```python
from build123d import *

# Parameters (mm, degrees)
BOSS_EXTRUDE1_DEPTH = 42
BOSS_EXTRUDE2_DEPTH = 1
BOSS_EXTRUDE3_DEPTH = 13


with BuildPart() as part:
    # Sketch1 → Boss-Extrude1 (new body)
    with BuildSketch(Plane(origin=(0, 0, 0), x_dir=(0, 0, -1), z_dir=(1, 0, 0))):
        Polygon((0, 4.2), (0, 0), (10.9, 0), (10.9, 0.81375), (1, 0.81375), (1, 1.91375), (0.9, 1.91375), (0.9, 3.2), (1, 3.2), (1, 4.2), align=None)
        Polygon((10.9, 0.81375), (10.9, 0), (21.8, 0), (21.8, 4.2), (20.8, 4.2), (20.8, 3.2), (20.9, 3.2), (20.9, 1.91375), (20.8, 1.91375), (20.8, 0.81375), align=None)
    extrude(amount=BOSS_EXTRUDE1_DEPTH)

    # Sketch2 → Boss-Extrude2 (add)
    with BuildSketch(Plane(origin=(42, 0, 0), x_dir=(0, 0, -1), z_dir=(1, 0, 0))):
        Polygon((0, 0), (21.8, 0), (21.8, 4.2), (16.8, 4.2), (16.8, 1.91375), (5, 1.91375), (5, 4.2), (0, 4.2), align=None)
    extrude(amount=BOSS_EXTRUDE2_DEPTH)

    # Sketch3 → Boss-Extrude3 (add)
    with BuildSketch(Plane.ZY):
        Polygon((-21.8, 4.2), (-21.8, 0), (0, 0), (0, 4.2), (-0.9, 4.2), (-0.9, 1.91375), (-1, 1.91375), (-1, 0.81375), (-20.8, 0.81375), (-20.8, 1.91375), (-20.9, 1.91375), (-20.9, 4.2), align=None)
    extrude(amount=BOSS_EXTRUDE3_DEPTH)


solid = part.part
```
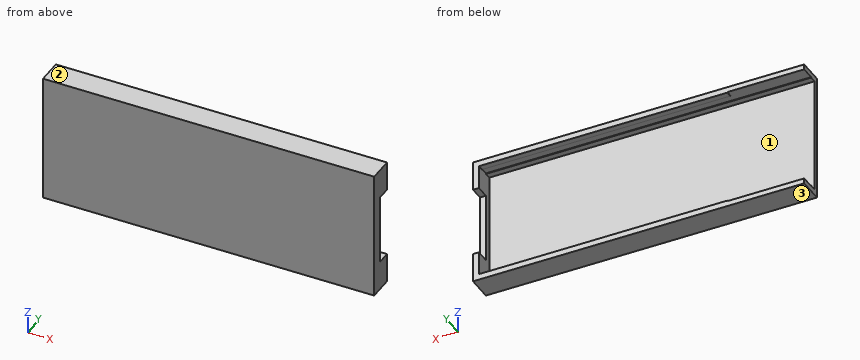
Check sheet for the modelled part. Datum: model origin and axes. Units: mm. Face numbers are marked on the shaded views. Round coordinates to 2 decimals unless told otherwise and drop trailing zeros. Order: outer loops, then holes, each group sorted by start corner. A loop starts at its lowest first (then second) coordinate and runs counter-clockwise, first axis right, second up. Notation, with made-up numbers: M 0,22.5 L 28,22.5 A17 ccw 28,38.5 Z; hole C 67.25,38.25 d1. An arc over 180 degrees is marked long. Answer in a Markdown table with one row per item.
(1) Section check B-B on z = -1.5. Record the boundary of the cut face in (x, y), plus the area to 3 significant figures.
Findings:
| item | result |
|---|---|
| outline | M -13,0 L 43,0 L 43,4.2 L 42,4.2 L 42,0.81 L -13,0.81 Z |
| area | 49.0 mm^2 |
(2) Section check C-C on x = 13. Record the boundary of the cut face in (y, z).
Findings:
| item | result |
|---|---|
| outline | M 0,-21.8 L 4.2,-21.8 L 4.2,-20.8 L 3.2,-20.8 L 3.2,-20.9 L 1.91,-20.9 L 1.91,-20.8 L 0.81,-20.8 L 0.81,-1 L 1.91,-1 L 1.91,-0.9 L 3.2,-0.9 L 3.2,-1 L 4.2,-1 L 4.2,0 L 0,0 Z |
(3) Draft check along Z on the marked faces 1, 2 and 3. Enter one of: +Z half, -Z half, draft (parallel to the pull), parting line (faces both ways), or undercut.
Findings:
| item | result |
|---|---|
| face 1 | undercut |
| face 2 | +Z half |
| face 3 | -Z half |
(4) Gauge pin test, flat ends, axial feed: pin 1 (1 mm diameter, centred on x = 24.5, z = -5.5, fed in from +Y); pin 2 (1.7 mm diameter, centred on y = 2, z = -7.5, fed in from -X). Record the tip position at first contact, or that the pin passes through.
Findings:
| item | result |
|---|---|
| pin 1 | stops at y = 0.81 |
| pin 2 | stops at x = 42 |
(5) Material ranges on line 1 along Z through (x, y) = (28.5, 1.25); line 2 along Z through (x, y) = (-8, 2.25); line 3 along X through (y, z) = (3.15, -3.5), recorded low to high. Write a range as from..to.
Findings:
| item | result |
|---|---|
| line 1 | z = -21.8..-20.8, -1..0 |
| line 2 | z = -21.8..-20.9, -0.9..0 |
| line 3 | x = 42..43 |
(6) Section check A-A on x = -8. Record the boundary of the cut face in (y, z).
Findings:
| item | result |
|---|---|
| outline | M 0,-21.8 L 4.2,-21.8 L 4.2,-20.9 L 1.91,-20.9 L 1.91,-20.8 L 0.81,-20.8 L 0.81,-1 L 1.91,-1 L 1.91,-0.9 L 4.2,-0.9 L 4.2,0 L 0,0 Z |
(7) Section check D-D on z = -6.5. Record the boundary of the cut face in (x, y), plus the area to 3 significant figures.
Findings:
| item | result |
|---|---|
| outline | M -13,0 L 43,0 L 43,1.91 L 42,1.91 L 42,0.81 L -13,0.81 Z |
| area | 46.7 mm^2 |
